Here's how the part is built. I have some questions about the finished solid (model axes, mm). Give positions to 0.01 mm unless a question says otherwise; leave off trailing zeros. Write each loop counter-clockwise with the first axis right and the second up, starting at its lowest first coordinate (ties: lowest second). Pieces come first, ordered by that corner, then holes. Notation, with made-up numbers: (55.5, 30) -> (59.5, 30) arc R23 ccw to (59.5, 56) -> close; hole circle Ø5 at (71, 81). An arc over 180 degrees is marked (long way). Use CSV: the item, a comma, the result in double quotes. Start each with the question number.
(1) I need wall thicknesses on L1, parallel to Y at x = 12.5, z = 2.3; L2, parallel to Y at x = 10.75, z = 1.1; L3, parallel to X at y = 47.5, z = 4.1. Which ranges of each line are inside material? Lowest first, please. Write a range as [from, to].
(2) Suppose I cut it at B-B on z = 2.65. List the corners of the cut face in (x, y) for me, plus the area to 3 significant figures.
(3) Suppose I cut it at C-C on x = 12.5. List the corners of the cut face in (y, z) for me.
(4) Suppose I cut it at A-A on y = 50. List the corners of the cut face in (x, z) for me.
(5) If we mould it in two halves opening along X, with no side actions, what happens to faces 1 (the cylindrical face through (10.1, 8.2, 2.5)), 2 (the flat face through (0, 59, 2)), 3 (the flat face through (12, 120, 2))? For each: pulls with the +X half, pulls with the -X half, needs draft (parallel to the pull), parting line crosses it, or undercut.
from build123d import *

# Parameters (mm, degrees)
SKETCH1_W           = 25
SKETCH1_H           = 120
SKETCH1_R           = 3
SKETCH1_R_2         = 8
BOSS_EXTRUDE1_DEPTH = 5
CHAMFER1_SIZE       = 1


with BuildPart() as part:
    # Sketch1 → Boss-Extrude1 (new body)
    with BuildSketch(Plane.XY):
        with Locations((12.5, 60)):
            Rectangle(SKETCH1_W, SKETCH1_H)
        with Locations((12.5, 110)):
            Circle(SKETCH1_R, mode=Mode.SUBTRACT)
        with Locations((12.5, 80)):
            Circle(SKETCH1_R_2, mode=Mode.SUBTRACT)
        with Locations((12.5, 50)):
            Circle(SKETCH1_R, mode=Mode.SUBTRACT)
        with Locations((12.5, 30)):
            Circle(SKETCH1_R, mode=Mode.SUBTRACT)
        with Locations((12.5, 10)):
            Circle(SKETCH1_R, mode=Mode.SUBTRACT)
    extrude(amount=BOSS_EXTRUDE1_DEPTH)

    # Chamfer1
    chamfer1_edges = [part.edges().sort_by_distance(p)[0] for p in [
        (4.5, 80, 0),
        (4.5, 80, 5),
    ]]
    chamfer(chamfer1_edges, length=CHAMFER1_SIZE)


solid = part.part
Geometry says:
1,L1,"[0, 7], [13, 27], [33, 47], [53, 72], [88, 107], [113, 120]"
1,L2,"[0, 7.56], [12.44, 27.56], [32.44, 47.56], [52.44, 72.19], [87.81, 107.56], [112.44, 120]"
1,L3,"[0, 10.84], [14.16, 25]"
2,outline,"(0, 0) -> (25, 0) -> (25, 120) -> (0, 120) -> close; hole circle Ø16 at (12.5, 80); hole circle Ø6 at (12.5, 10); hole circle Ø6 at (12.5, 30); hole circle Ø6 at (12.5, 50); hole circle Ø6 at (12.5, 110)"
2,area,"2,690 mm²"
3,outline,"(0, 0) -> (7, 0) -> (7, 5) -> (0, 5) -> close; (13, 0) -> (27, 0) -> (27, 5) -> (13, 5) -> close; (33, 0) -> (47, 0) -> (47, 5) -> (33, 5) -> close; (53, 0) -> (71, 0) -> (72, 1) -> (72, 4) -> (71, 5) -> (53, 5) -> close; (88, 1) -> (89, 0) -> (107, 0) -> (107, 5) -> (89, 5) -> (88, 4) -> close; (113, 0) -> (120, 0) -> (120, 5) -> (113, 5) -> close"
4,outline,"(0, 0) -> (9.5, 0) -> (9.5, 5) -> (0, 5) -> close; (15.5, 0) -> (25, 0) -> (25, 5) -> (15.5, 5) -> close"
5,face 1,"undercut"
5,face 2,"pulls with the -X half"
5,face 3,"needs draft"
